Geometry check sheet. Reference: drawing and pictorial views, mm from the part's lowest x, y, z. A direction names the side the tool comes from. Give positions to 0.01 mm unless a question says otherwise; leave off trailing zeros. Write each loop counter-clockwise with the first axis right and the second up, starting at its lowest first coordinate (ties: lowest second). Pieces come first, ordered by that corner, then holes.
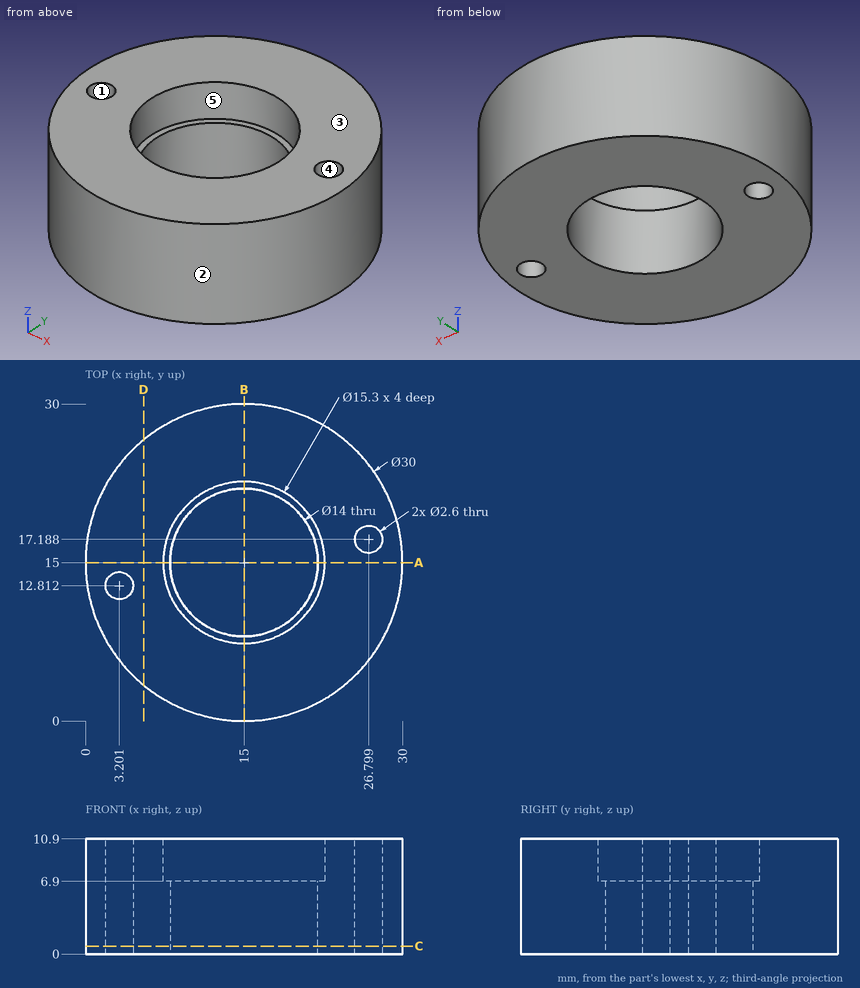
Item 1: Depth check by flat-ended pin: pin 1 (4 mm diameter, centred on y = 23, z = 2.5, fed in from +X); pin 2 (4.5 mm diameter, centred on x = 14, y = 18, fed in from +Z); pin 3 (4 mm diameter, centred on x = 18.5, z = 8, fed in from -Y) (3 decimals); pin 4 (1 mm diameter, centred on x = 21, z = 9.5, fed in from -Y) (1 decimal). Enter the tip coordinate at first touch or a pass-through.
Answer key:
pin 1: stops at x = 28.75
pin 2: passes through
pin 3: stops at y = 0.075
pin 4: stops at y = 1
Item 2: Release check for a two-part mould opening along Y. For the marked faces 1, 2 and 3 record: released by +Y, released by -Y, zero draft, split by the parting line, or undercut.
Answer key:
face 1: undercut
face 2: split by the parting line
face 3: zero draft
Item 3: Sectioned sample at D-D on x = 5.5. Record the cut outline in (y, z).
Answer key:
outline: (3.39, 0) - (26.61, 0) - (26.61, 10.9) - (3.39, 10.9) - close
Item 4: Set-up check for the marked faces 4 and 5: record each of +Z, -Z, +X, -X, +Y, -Y from which the full face is reachable in a straight line by a thin tool's end or side.
Answer key:
face 4: +Z, -Z
face 5: +Z
Item 5: Scan lines: line 1 along Y through (x, z) = (15, 5); line 2 along Y through (x, z) = (21.25, 9) (1 decimal); line 3 along X through (y, z) = (17.25, 10). Record each from-to range of solid material in increasing order.
Answer key:
line 1: y = 0 to 8, 22 to 30
line 2: y = 1.4 to 10.6, 19.4 to 28.6
line 3: x = 0.17 to 7.69, 22.31 to 25.5, 28.1 to 29.83
Item 6: Sectioned sample at A-A on y = 15. Record the cut outline in (x, z), then the cut area to 3 significant figures.
Answer key:
outline: (0, 0) - (8, 0) - (8, 6.9) - (7.35, 6.9) - (7.35, 10.9) - (0, 10.9) - close; (22, 0) - (30, 0) - (30, 10.9) - (22.65, 10.9) - (22.65, 6.9) - (22, 6.9) - close
area: 169 mm2
Item 7: Sectioned sample at C-C on z = 0.75. Record the cut outline in (x, y), then the cut area to 3 significant figures.
Answer key:
outline: circle Ø30 at (15, 15); hole circle Ø2.6 at (3.2, 12.81); hole circle Ø14 at (15, 15); hole circle Ø2.6 at (26.8, 17.19)
area: 542 mm2
